The listing builds one solid part. Answer for the finished solid, in the listing's coordinates (mm). Round coordinates to 2 decimals unless told otherwise and drop trailing zeros. Order: outer loops, then holes, each group sorted by start corner. A loop starts at its lowest first (then second) coordinate and runs counter-clockwise, first axis right, second up. Notation, with made-up numbers: M 62,39 L 95,39 A28 ccw 95,69 Z; hole C 66,29.25 d4. An arc over 180 degrees is marked long. Put each result on its own line as item: value. Start each with the question number.
1. Consider line 1 (Y direction, x = 130, z = -0.75); line 2 (Y direction, x = 61.5, z = -1.5); line 3 (X direction, y = 209.5, z = -1). Determine where each line is inside the solid, lowest interval first.
2. The part is cut by section C-C (x = 221). Give the vertices of the cut face in (y, z).
3. The part is cut by section B-B (y = 166.5). Give the vertices of the cut face in (x, z), then the cut area to 3 significant figures.
4. The part is cut by section A-A (x = 88). Give the vertices of the cut face in (y, z).
5. The part is cut by section D-D (z = -1.25). Count the separate pieces of the cut face and the enclosed holes in it, then the cut area to 3 significant figures.
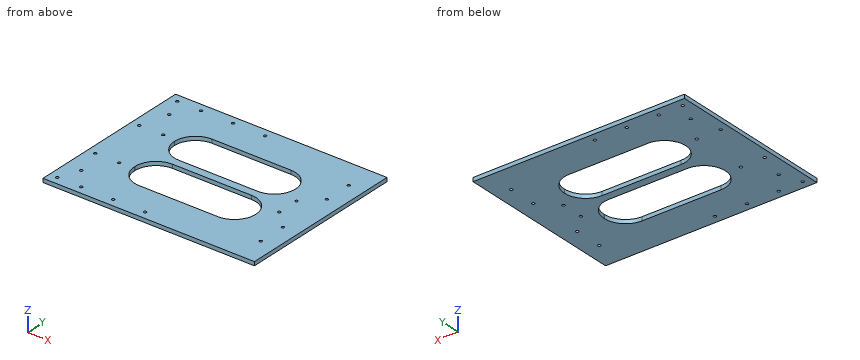
Autodesk Inventor part; units mm, degrees
ref_plane "YZ Plane" through (0, 0, 0) normal (1, 0, 0) x (0, 1, 0)
ref_plane "XZ Plane" through (0, 0, 0) normal (0, 1, 0) x (-1, 0, 0)
ref_plane "XY Plane" through (0, 0, 0) normal (0, 0, 1) x (1, 0, 0)
ref_plane "Work Plane1" through (0, 0, 0) normal (0, 0, 1) x (1, 0, 0)
sketch "Sketch1" plane through (0, 0, 0) normal (0, 0, 1) x (1, 0, 0)
  line L0 (0, 273.904) -> (158.3386, 273.904)
  line L1 (133.9788, 273.904) -> (133.9788, 6.096)
  line L2 (-34.2962, 6.096) -> (302.2538, 6.096)
  line L3 (302.2538, 6.096) -> (302.2538, 273.904)
  line L4 (302.2538, 273.904) -> (-34.2962, 273.904)
  line L5 (-34.2962, 273.904) -> (-34.2962, 6.096)
  line L6 (-34.2962, 6.096) -> (302.2538, 273.904) construction
  line L7 (302.2538, 6.096) -> (-34.2962, 273.904) construction
  point P0 (0, 0)
  point P1 (0, 6.096)
  point P2 (133.9788, 140)
  dimension "d0" = 336.55
extrude "Extrusion1" add sketch "Sketch1" against normal blind 6.096
sketch "Sketch2" plane through (0, 0, -6.096) normal (0, 0, -1) x (-1, 0, 0)
  line L0 (-302.2538, 6.096) -> (34.2962, 6.096)
  line L1 (34.2962, 6.096) -> (34.2962, 273.904)
  line L2 (34.2962, 273.904) -> (-302.2538, 273.904)
  line L3 (-302.2538, 273.904) -> (-302.2538, 6.096)
  line L4 (34.2962, 6.096) -> (-16.5038, 6.096)
  line L5 (-302.2538, 6.096) -> (34.2962, 6.096)
  line L6 (-16.5038, 6.096) -> (-67.3038, 6.096)
  line L7 (-67.3038, 6.096) -> (-118.1038, 6.096)
  line L8 (-16.5038, 6.096) -> (-16.5038, 18.796)
  circle A0 centre (-16.5038, 18.796) radius 2.2225
  circle A1 centre (-118.1038, 18.796) radius 2.2225
  circle A2 centre (-67.3038, 18.796) radius 2.2225
  line L9 (-16.5038, 18.796) -> (21.5962, 18.796)
  circle A3 centre (21.5962, 18.796) radius 2.2225
  line L10 (34.2962, 6.096) -> (34.2962, 273.904)
  line L11 (34.2962, 140) -> (8.8962, 140)
  line L12 (34.2962, 273.904) -> (-16.5038, 273.904)
  line L13 (-16.5038, 273.904) -> (-67.3038, 273.904)
  line L14 (-67.3038, 273.904) -> (-118.1038, 273.904)
  line L15 (-16.5038, 273.904) -> (-16.5038, 261.204)
  circle A4 centre (-16.5038, 261.204) radius 2.2225
  circle A5 centre (-118.1038, 261.204) radius 2.2225
  circle A6 centre (-67.3038, 261.204) radius 2.2225
  line L16 (-16.5038, 261.204) -> (21.5962, 261.204)
  circle A7 centre (21.5962, 261.204) radius 2.2225
  point P0 (0, 0)
  point P1 (0, 280)
  dimension "d3" = 50.8
  dimension "d4" = 50.8
  dimension "d5" = 50.8
  dimension "d6" = 12.7
  dimension "d7" = 4.445
  dimension "d8" = 4.445
  dimension "d9" = 4.445
  dimension "d10" = 38.1
  dimension "d11" = 4.445
extrude "Extrusion2" cut sketch "Sketch2" against normal blind 10.8585 contours A3 | A0 L9 L8 | L8 L9 A0 | A7 | A4 L16 L15 | L15 L16 A4 | A1 | A2 | A5 | A6
sketch "Sketch3" plane through (0, 0, -6.096) normal (0, 0, -1) x (-1, 0, 0)
  circle A0 centre (-67.3038, 261.204) radius 2.2225
  circle A1 centre (21.5962, 261.204) radius 2.2225
  circle A2 centre (-67.3038, 18.796) radius 2.2225
  circle A3 centre (-16.5038, 18.796) radius 2.2225
  circle A4 centre (-118.1038, 18.796) radius 2.2225
  circle A5 centre (21.5962, 18.796) radius 2.2225
  circle A6 centre (-16.5038, 261.204) radius 2.2225
  circle A7 centre (-118.1038, 261.204) radius 2.2225
  line L0 (-302.2538, 6.096) -> (34.2962, 6.096)
  line L1 (34.2962, 6.096) -> (34.2962, 273.904)
  line L2 (34.2962, 273.904) -> (-302.2538, 273.904)
  line L3 (-302.2538, 273.904) -> (-302.2538, 6.096)
  circle A8 centre (8.8962, 228.9) radius 2.2225
  circle A9 centre (21.5962, 184.45) radius 2.2225
  circle A10 centre (-16.5038, 184.45) radius 2.2225
  circle A11 centre (-16.5038, 95.55) radius 2.2225
  circle A12 centre (8.8962, 51.1) radius 2.2225
  circle A13 centre (21.5962, 95.55) radius 2.2225
  point P0 (0, 0)
  dimension "d20" = 4.445
  dimension "d21" = 4.445
  dimension "d22" = 4.445
  dimension "d23" = 4.445
  dimension "d24" = 4.445
  dimension "d25" = 4.445
extrude "Extrusion3" cut sketch "Sketch3" against normal blind 10.8585 contours A8 | A9 | A10 | A11 | A12 | A13
sketch "Sketch4" plane through (0, 0, -6.096) normal (0, 0, -1) x (-1, 0, 0)
  circle A0 centre (8.8962, 51.1) radius 2.2225
  circle A1 centre (-16.5038, 184.45) radius 2.2225
  circle A2 centre (8.8962, 228.9) radius 2.2225
  circle A3 centre (21.5962, 184.45) radius 2.2225
  circle A4 centre (-16.5038, 95.55) radius 2.2225
  circle A5 centre (21.5962, 95.55) radius 2.2225
  circle A6 centre (-67.3038, 261.204) radius 2.2225
  circle A7 centre (21.5962, 261.204) radius 2.2225
  circle A8 centre (-67.3038, 18.796) radius 2.2225
  circle A9 centre (-16.5038, 18.796) radius 2.2225
  circle A10 centre (-118.1038, 18.796) radius 2.2225
  circle A11 centre (21.5962, 18.796) radius 2.2225
  circle A12 centre (-16.5038, 261.204) radius 2.2225
  circle A13 centre (-118.1038, 261.204) radius 2.2225
  line L0 (-302.2538, 6.096) -> (34.2962, 6.096)
  line L1 (34.2962, 6.096) -> (34.2962, 273.904)
  line L2 (34.2962, 273.904) -> (-302.2538, 273.904)
  line L3 (-302.2538, 273.904) -> (-302.2538, 6.096)
  line L4 (-302.2538, 6.096) -> (-302.2538, 273.904)
  line L5 (-302.2538, 228.9) -> (-276.8538, 228.9) construction
  line L6 (-302.2538, 140) -> (-241.6696, 140)
  circle A14 centre (-276.8538, 228.9) radius 2.2225
  circle A15 centre (-276.8538, 184.45) radius 2.2225
  circle A16 centre (-276.8538, 95.55) radius 2.2225
  circle A17 centre (-276.8538, 51.1) radius 2.2225
  line L7 (-276.8538, 184.45) -> (-238.7538, 184.45) construction
  circle A18 centre (-249.9131, 157.5092) radius 2.2225
  circle A19 centre (-249.9131, 122.4908) radius 2.2225
  point P0 (0, 0)
  dimension "d31" = 4.445
  dimension "d32" = 4.445
  dimension "d33" = 4.445
  dimension "d37" = 4.445
  dimension "d38" = 4.445
extrude "Extrusion4" cut sketch "Sketch4" against normal blind 10.8585 contours A14 | A15 | A16 | A17 | A18 | A19
sketch "Sketch5" plane through (0, 0, 0) normal (0, 0, 1) x (1, 0, 0)
  line L0 (253.9788, 60) -> (13.9788, 60)
  line L1 (13.9788, 60) -> (13.9788, 220)
  line L2 (13.9788, 220) -> (253.9788, 220)
  line L3 (253.9788, 220) -> (253.9788, 60)
  line L4 (37.6584, 66.1088) -> (230.2993, 66.1088)
  line L5 (230.2993, 66.1088) -> (230.2993, 213.8912)
  line L6 (230.2993, 213.8912) -> (37.6584, 213.8912)
  line L7 (37.6584, 213.8912) -> (37.6584, 66.1088)
  line L8 (37.6584, 66.1088) -> (230.2993, 213.8912) construction
  line L9 (230.2993, 66.1088) -> (37.6584, 213.8912) construction
  point P0 (0, 0)
  point P1 (133.9788, 140)
extrude "Extrusion5" cut sketch "Sketch5" against normal blind 10.8585 contours L7 L6 L5 L4
sketch "Sketch6" plane through (0, 0, 0) normal (0, 0, 1) x (1, 0, 0)
  line L0 (28.0721, 134.0106) -> (240.3993, 134.0106)
  line L1 (240.3993, 134.0106) -> (240.3993, 146.7106)
  line L2 (240.3993, 146.7106) -> (28.0721, 146.7106)
  line L3 (28.0721, 146.7106) -> (28.0721, 134.0106)
  line L4 (28.0721, 134.0106) -> (240.3993, 146.7106) construction
  line L5 (240.3993, 134.0106) -> (28.0721, 146.7106) construction
  point P0 (0, 0)
  point P1 (134.2357, 140.3606)
  dimension "d43" = 12.7
extrude "Extrusion6" add sketch "Sketch6" against normal up to surface (6.096 mm away)
fillet "Fillet1" radius 33.5534 8 edges at (230.2993, 66.1088, -3.048) (230.2993, 134.0106, -3.048) (230.2993, 146.7106, -3.048) (230.2993, 213.8912, -3.048) (37.6584, 66.1088, -3.048) (37.6584, 134.0106, -3.048) (37.6584, 146.7106, -3.048) (37.6584, 213.8912, -3.048)
properties part number "BasePlate"
Resolved:
1. line 1: 6.1 to 66.11, 134.01 to 146.71, 213.89 to 273.9
1. line 2: 6.1 to 67.55, 132.57 to 148.15, 212.45 to 273.9
1. line 3: -34.3 to 54.62, 213.34 to 302.25
2. outline: M 6.1,-6.1 L 76.48,-6.1 L 76.48,0 L 6.1,0 Z; M 123.64,-6.1 L 157.08,-6.1 L 157.08,0 L 123.64,0 Z; M 203.52,-6.1 L 273.9,-6.1 L 273.9,0 L 203.52,0 Z
3. outline: M -34.3,-6.1 L 40.61,-6.1 L 40.61,0 L -34.3,0 Z; M 227.35,-6.1 L 302.25,-6.1 L 302.25,0 L 227.35,0 Z
3. area: 913 mm2
4. outline: M 6.1,-6.1 L 66.11,-6.1 L 66.11,0 L 6.1,0 Z; M 134.01,-6.1 L 146.71,-6.1 L 146.71,0 L 134.01,0 Z; M 213.89,-6.1 L 273.9,-6.1 L 273.9,0 L 213.89,0 Z
5. separate pieces: 1
5. enclosed holes: 22
5. area: 65,700 mm2
